from build123d import *

# Parameters (mm, degrees)
F1_DEPTH = 2.38125
F2_R     = 2.38125
F3_DEPTH = 2.38225
F5_DEPTH = 25.4


# Not quite as in the source:
# - a length typed as a fraction of an inch, garbled in the dataset ("3 / 203.2 mm" for 3/8 in), is restored


with BuildPart() as f1:
    # F0 (on Front) → F1 (new body)
    with BuildSketch(Plane.XZ):
        with BuildLine():
            Line((60.325, 19.05), (7.9375, 19.05))
            ThreePointArc((7.9375, 19.05), (2.3248399243, 16.7251600757), (0, 11.1125))
            Line((0, 11.1125), (0, 0))
            Line((0, 0), (9.525, 0))
            Line((9.525, 0), (12.1173647876, 7.6271664624))
            ThreePointArc((12.1173647876, 7.6271664624), (13.4786145605, 9.5135918491), (15.6631963617, 10.3130942181))
            Line((15.6631963617, 10.3130942181), (60.325, 12.7))
            Line((60.325, 12.7), (60.325, 19.05))
        make_face()
    extrude(amount=F1_DEPTH)

    # F2 (on face) → F3 (cut, through all)
    with BuildSketch(Plane.XZ.offset(2.38125)):
        with Locations((7.9375, 11.1125)):
            Circle(F2_R)
    extrude(amount=-F3_DEPTH, mode=Mode.SUBTRACT)

    # F4 (on face) → F5 (cut)
    with BuildSketch(Plane.XY.offset(19.05)):
        Polygon((60.325, 0), (47.2817567568, 0), (60.325, -0.79375), align=None)
        Polygon((60.325, -2.38125), (60.325, -1.5875), (47.2817567568, -2.38125), align=None)
    extrude(amount=-F5_DEPTH, mode=Mode.SUBTRACT)


solid = f1.part
Build history of the part. All positions in model axes, mm. Give positions to 0.01 mm unless a question says otherwise; leave off trailing zeros. Loops run counter-clockwise (first coordinate to the right, second up) from the corner with the lowest first, then second, coordinate; pieces in that order, holes last. Notation, with made-up numbers: (18, -2.5) - (67, -2.5) arc R29 cw to (67, 29.5) - close; hole circle Ø2 at (89.25, 11.25). An arc over 180 degrees is marked (long way). Write item = value, one per line. Start each with the question number.
1) Band-saw the part on D-D on x = 38. Give the cut face in (y, z).
2) Band-saw the part on C-C on x = 30. Give the cut face in (y, z), plus the area to 3 significant figures.
3) Band-saw the part on A-A on z = 9.25. Give the cut face in (x, y).
4) Drop flat-ended pins along their axis: pin 1 Ø10 at (x, z) = (40, 14.5) entering from +Y; pin 2 Ø1.5 at (x, z) = (26.5, 9.5) entering from -Y. Give the stop position or say it passes through.
5) Probe probe 1 along Z at (x, y) = (7, -2.1); probe 2 along Z at (x, y) = (9, -0.6); probe 3 along Z at (x, y) = (20.5, -1). List the from-to ranges inside material, lowest first. Write a range as from..to.
6) Band-saw the part on B-B on z = 14.25. Give the cut face in (x, y) (1 decimal), plus the area to 3 significant figures.
7) Pull direction Z, two halves, no side cores. Call faces 1 (the cylindrical face through (6.18, -1.21, 12.72)), 2 (the flat face through (5, -1, 0)), 3 (the flat face through (18, 0, 12)): +Z half, -Z half, draft (parallel to the pull), parting line (faces both ways), or undercut.
Final values:
q1.outline = (-2.38, 11.51) - (0, 11.51) - (0, 19.05) - (-2.38, 19.05) - close
q2.outline = (-2.38, 11.08) - (0, 11.08) - (0, 19.05) - (-2.38, 19.05) - close
q2.area = 19.0 mm²
q3.outline = (0, -2.38) - (6.45, -2.38) - (6.45, 0) - (0, 0) - close; (9.42, -2.38) - (13.17, -2.38) - (13.17, 0) - (9.42, 0) - close
q4.pin_1 = 0
q4.pin_2 = through
q5.probe_1 = 0..8.92, 13.3..18.99
q5.probe_2 = 0..8.98, 13.24..19.05
q5.probe_3 = 10.57..19.05
q6.outline = (0.6, -2.4) - (47.3, -2.4) - (60.3, -1.6) - (60.3, -0.8) - (47.3, 0) - (0.6, 0) - close
q6.area = 132 mm²
q7.face_1 = undercut
q7.face_2 = -Z half
q7.face_3 = draft
